Here's the drawing with two shaded views (mm, measured from the low corner). I have some questions. A direction names the side the tool comes from. Give positions to 0.01 mm unless a question says otherwise; leave off trailing zeros. Write each loop counter-clockwise with the first axis right and the second up, starting at its lowest first coordinate (ties: lowest second). Pieces come first, ordered by that corner, then holes. Notation, with made-up numbers: (35.25, 59.5) - (63.25, 59.5) arc R26 ccw to (63.25, 97.5) - close; hole circle Ø1 at (46, -18). An arc over 180 degrees is marked (long way). Answer as CSV lines item,"result". Start each with the question number.
Q1. Will these pins go through, and if not, where does the flat tip stop? pin 1 Ø2 at (x, z) = (2.5, 2) entering from -Y; pin 2 Ø3 at (x, z) = (1.5, 1) entering from +Y.
Q2. Imagine slicing it at D-D on y = 3.15. List the corners of the cut face in (x, z) for me (3 decimals), and give its area (4 significant figures).
Q3. Imagine slicing it at B-B on y = 1.1. List the corners of the cut face in (x, z) for me, and give its area (3 significant figures).
Q4. We'd pull the mould along X, two halves only. Please class the marked faces 1, 2 and 3: pulls with the +X half, pulls with the -X half, needs draft (parallel to the pull), parting line crosses it, or undercut.
Q5. Imagine slicing it at C-C on z = 1.25. List the corners of the cut face in (x, y) for me, and give its area (3 significant figures).
Q6. Imagine slicing it at A-A on y = 0.45. List the corners of the cut face in (x, z) for me.
Q7. If I drill on line 1 along X through (y, z) = (1.65, 4.4); line 2 along Z through (x, y) = (5, 4.15) (3 decimals); line 3 along Z through (x, y) = (1.25, 3.55), over which ranges is the centre line in solid material (lowest first)?
Q8. On a 3-axis mill with a long thin cutter (end or side, diameter ignored), from which of +Z, -Z, +X, -X, +Y, -Y can I reach the whole of each face in a straight line? I mean the marked faces 4, 5, 6 and 7. Say none if no direction works.
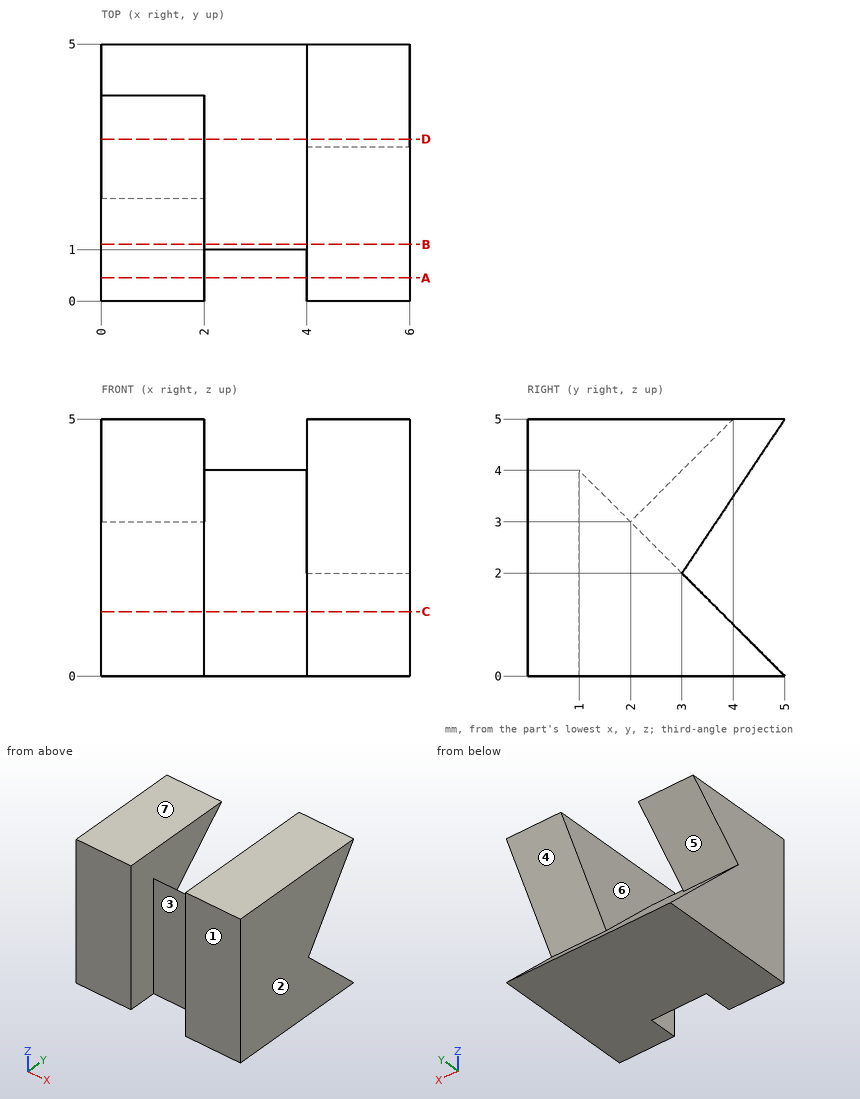
Conclusion:
1,pin 1,"y = 0"
1,pin 2,"y = 5"
2,outline,"(0, 0) - (6, 0) - (6, 1.85) - (0, 1.85) - close; (0, 4.15) - (2, 4.15) - (2, 5) - (0, 5) - close; (4, 2.225) - (6, 2.225) - (6, 5) - (4, 5) - close"
2,area,"18.35 mm^2"
3,outline,"(0, 0) - (6, 0) - (6, 5) - (4, 5) - (4, 3.9) - (2, 3.9) - (2, 5) - (0, 5) - close"
3,area,"27.8 mm^2"
4,face 1,"needs draft"
4,face 2,"pulls with the +X half"
4,face 3,"undercut"
5,outline,"(0, 0) - (2, 0) - (2, 1) - (4, 1) - (4, 0) - (6, 0) - (6, 3.75) - (0, 3.75) - close"
5,area,"20.5 mm^2"
6,outline,"(0, 0) - (2, 0) - (2, 5) - (0, 5) - close; (4, 0) - (6, 0) - (6, 5) - (4, 5) - close"
7,line 1,"0 to 2, 4 to 6"
7,line 2,"0 to 0.85, 3.725 to 5"
7,line 3,"0 to 1.45, 4.55 to 5"
8,face 4,"+X, -X, +Y"
8,face 5,"-X, +Y"
8,face 6,"+Z"
8,face 7,"+Z, +X, -X, +Y, -Y"
